from build123d import *

# Parameters (mm, degrees)
ESQUISSE1_W             = 48
ESQUISSE1_H             = 273
BOSS_EXTRU_1_DEPTH      = 24
ENL_V_MAT_EXTRU_1_DEPTH = 147.670549191
ESQUISSE5_R             = 4.5
ENL_V_MAT_EXTRU_2_DEPTH = 141.656496473


with BuildPart() as part:
    # Esquisse1 → Boss.-Extru.1 (new body)
    with BuildSketch(Plane.XY):
        Rectangle(ESQUISSE1_W, ESQUISSE1_H)
    extrude(amount=BOSS_EXTRU_1_DEPTH)

    # Esquisse4 → Enlèv. mat.-Extru.1 (cut, through all)
    with BuildSketch(Plane(origin=(24, 0, 0), x_dir=(0, 0, -1), z_dir=(1, 0, 0))):
        Polygon((-24, -136.5), (0, -62.635595108), (0, -136.5), align=None)
    extrude(amount=-ENL_V_MAT_EXTRU_1_DEPTH, mode=Mode.SUBTRACT)

    # Esquisse5 → Enlèv. mat.-Extru.2 (cut, through all)
    with BuildSketch(Plane.XY.offset(24)):
        with Locations((0, 112.5)):
            Circle(ESQUISSE5_R)
    extrude(amount=-ENL_V_MAT_EXTRU_2_DEPTH, mode=Mode.SUBTRACT)


solid = part.part
Verification items for the finished model (mm, model axes). Give positions to 0.01 mm unless a question says otherwise; leave off trailing zeros. Order: outer loops, then holes, each group sorted by start corner. A loop starts at its lowest first (then second) coordinate and runs counter-clockwise, first axis right, second up. Notation, with made-up numbers: (-15.75, -17) -> (33.25, -17) arc R33 cw to (33.25, 17) -> close; hole circle Ø8 at (76, 66). An arc over 180 degrees is marked (long way). Answer as CSV lines item,"result".
Q1. Release check for a two-part mould opening along X. For faces 1 (the flat face through (24, 28, 12)), 2 (the flat face through (0, 136.5, 12)), 3 (the cylindrical face through (-0.59, 116.96, 12.17)) record: +X half, -X half, draft (parallel to the pull), parting line (faces both ways), or undercut.
Solutions:
face 1,"+X half"
face 2,"draft"
face 3,"undercut"
Q2. Depth check by flat-ended pin: pin 1 (14.5 mm diameter, centred on x = 0, y = 112.5, fed in from -Z); pin 2 (3 mm diameter, centred on x = 14, y = -104, fed in from -Z); pin 3 (8 mm diameter, centred on x = 14, y = -85, fed in from -Z). Enter the tip coordinate at first touch or a pass-through.
Solutions:
pin 1,"stops at z = 0"
pin 2,"stops at z = 12.95"
pin 3,"stops at z = 5.97"
Q3. Sectioned sample at A-A on y = 112.5. Record the cut outline in (x, z), plus the area to 3 significant figures.
Solutions:
outline,"(-24, 0) -> (-4.5, 0) -> (-4.5, 24) -> (-24, 24) -> close; (4.5, 0) -> (24, 0) -> (24, 24) -> (4.5, 24) -> close"
area,"936 mm²"
Q4. Sectioned sample at D-D on x = 16. Record the cut outline in (y, z).
Solutions:
outline,"(-136.5, 24) -> (-62.64, 0) -> (136.5, 0) -> (136.5, 24) -> close"
Q5. Sectioned sample at B-B on x = 0. Record the cut outline in (y, z), plus the area to 3 significant figures.
Solutions:
outline,"(-136.5, 24) -> (-62.64, 0) -> (108, 0) -> (108, 24) -> close; (117, 0) -> (136.5, 0) -> (136.5, 24) -> (117, 24) -> close"
area,"5,450 mm²"
Q6. Sectioned sample at C-C on z = 14.75. Record the cut outline in (x, y).
Solutions:
outline,"(-24, -108.03) -> (24, -108.03) -> (24, 136.5) -> (-24, 136.5) -> close; hole circle Ø9 at (0, 112.5)"
Q7. Scan lines: probe 1 along Z at (x, y) = (4, -122); probe 2 along Z at (x, y) = (-21, -100.5). Record each from-to range of solid material in increasing order.
Solutions:
probe 1,"z = 19.29 to 24"
probe 2,"z = 12.3 to 24"
